Could you check a few things on this model? Use its own coordinates, in mm. A direction names the side the tool comes from. Coordinates: 2 decimals unless noted, no trailing zeros. Write each loop counter-clockwise with the first axis right and the second up, starting at its lowest first coordinate (ties: lowest second). Pieces come first, ordered by that corner, then holes. Notation, with made-up numbers: (-21, 43.25) - (-5, 43.25) arc R17 ccw to (-5, 52.25) - close; hole circle Ø2 at (61.25, 76.5). An arc over 180 degrees is marked (long way). Answer as a JSON object with one key per item and string values. Group by question number.
1) If we section it at C-C (z = 93): Write out the boundary of the cut face in (x, y), plus the area to 3 significant figures.
2) Please list where these lines run through material, in increasing order: line 1 along Z through (x, y) = (-20, 13.5); line 2 along Y through (x, z) = (-0.5, 97); line 3 along X through (y, z) = (-2, 117).
3) If we section it at A-A (y = 0): Write out the boundary of the cut face in (x, z).
4) On a 3-axis mill with a long thin cutter (end or side, diameter ignored), from which of +Z, -Z, +X, -X, +Y, -Y can I reach the whole of each face in a straight line? I mean faces 1 (the cylindrical face through (-1.08, -4.88, 114.44)), 2 (the cylindrical face through (-1.08, 4.88, -87.32)), 3 (the flat face through (0, 0, 155)). Say none if no direction works.
5) If we section it at D-D (y = -18): Write out the boundary of the cut face in (x, z).
6) Will these pins go through, and if not, where does the flat tip stop? pin 1 Ø3 at (x, y) = (13, -17.5) entering from +Z; pin 2 Ø12 at (y, z) = (10, 109.5) entering from +X; pin 3 Ø10 at (x, z) = (-13.5, 97.5) entering from +Y; pin 4 Ø4 at (y, z) = (4.5, 102) entering from -X.
```python
from build123d import *

# Parameters (mm, degrees)
F0_W     = 50
F0_H     = 50
F1_DEPTH = 75
F2_R     = 5
F3_DEPTH = 80
F4_R     = 5
F5_DEPTH = 25


with BuildPart() as f1:
    # F0 (on Top) → F1 (new body, symmetric)
    with BuildSketch(Plane.XY):
        Rectangle(F0_W, F0_H)
    extrude(amount=F1_DEPTH, both=True)

    # F2 (on face) → F3 (join)
    with BuildSketch(Plane.XY.offset(75)):
        Circle(F2_R)
    extrude(amount=F3_DEPTH)

    # F4 (on face) → F5 (join)
    with BuildSketch(Plane(origin=(0, 0, -75), x_dir=(1, 0, 0), z_dir=(0, 0, -1))):
        Circle(F4_R)
    extrude(amount=F5_DEPTH)


solid = f1.part
```
Here are the results:
{
 "1": {"outline": "circle Ø10 at (0, 0)", "area": "78.5 mm²"},
 "2": {"line 1": "z = -75 to 75", "line 2": "y = -4.97 to 4.97", "line 3": "x = -4.58 to 4.58"},
 "3": {"outline": "(-25, -75) - (-5, -75) - (-5, -100) - (5, -100) - (5, -75) - (25, -75) - (25, 75) - (5, 75) - (5, 155) - (-5, 155) - (-5, 75) - (-25, 75) - close"},
 "4": {"face 1": "+Z", "face 2": "-Z", "face 3": "+Z, +X, -X, +Y, -Y"},
 "5": {"outline": "(-25, -75) - (25, -75) - (25, 75) - (-25, 75) - close"},
 "6": {"pin 1": "stops at z = 75", "pin 2": "stops at x = 3", "pin 3": "passes through", "pin 4": "stops at x = -4.33"}
}
